```python
from build123d import *

# Parameters (mm, degrees)
SKETCH1_W           = 31.75
SKETCH1_H           = 3.175
BOSS_EXTRUDE1_DEPTH = 31.75
BOSS_EXTRUDE2_DEPTH = 31.75
SKETCH3_W           = 5.08
SKETCH3_H           = 10.541
BOSS_EXTRUDE3_DEPTH = 31.75
SKETCH4_R           = 2.2463125
SKETCH4_R_2         = 2.1193125
CUT_EXTRUDE1_DEPTH  = 31.75
SKETCH6_R           = 2.1193125
BOSS_EXTRUDE4_DEPTH = 15.875
FILLET1_R           = 0.762


with BuildPart() as part:
    # Sketch1 → Boss-Extrude1 (new body)
    with BuildSketch(Plane(origin=(0, 0, 0), x_dir=(1, 0, 0), z_dir=(0, 1, 0))):
        Rectangle(SKETCH1_W, SKETCH1_H)
    extrude(amount=BOSS_EXTRUDE1_DEPTH)

    # Sketch2 → Boss-Extrude2 (add)
    with BuildSketch(Plane(origin=(0, 31.75, 0), x_dir=(1, 0, 0), z_dir=(0, 1, 0))):
        with BuildLine():
            Line((-15.875, 1.5875), (-15.875, 12.3825))
            Line((-15.875, 12.3825), (-10.795, 12.3825))
            ThreePointArc((-10.795, 12.3825), (-7.633217703, 4.749282297), (0, 1.5875))
            Line((0, 1.5875), (-15.875, 1.5875))
        make_face()
    boss_extrude2 = extrude(amount=-BOSS_EXTRUDE2_DEPTH)

    # Mirror1: Boss-Extrude2 across plane
    add(boss_extrude2.mirror(Plane(origin=(0, 0, 0), x_dir=(0, 0, 1), z_dir=(1, 0, 0))))

    # Sketch3 → Boss-Extrude3 (add)
    with BuildSketch(Plane(origin=(0, 31.75, 0), x_dir=(1, 0, 0), z_dir=(0, 1, 0))):
        with Locations((-13.335, 17.653)):
            Rectangle(SKETCH3_W, SKETCH3_H)
    boss_extrude3 = extrude(amount=-BOSS_EXTRUDE3_DEPTH)

    # Mirror2: Boss-Extrude3 across plane
    add(boss_extrude3.mirror(Plane(origin=(0, 0, 0), x_dir=(0, 0, 1), z_dir=(1, 0, 0))))

    # Sketch4 → Cut-Extrude1 (cut)
    with BuildSketch(Plane.XY.offset(1.5875)):
        with Locations((0, 26.035)):
            Circle(SKETCH4_R)
        with Locations((0, 5.715)):
            Circle(SKETCH4_R_2)
    extrude(amount=-CUT_EXTRUDE1_DEPTH, mode=Mode.SUBTRACT)

    # Sketch6 → Boss-Extrude4 (add)
    with BuildSketch(Plane.XY.offset(1.5875)):
        with Locations((0, 5.715)):
            Circle(SKETCH6_R)
    extrude(amount=-BOSS_EXTRUDE4_DEPTH)

    # Fillet1
    fillet1_edges = [part.edges().sort_by_distance(p)[0] for p in [
        (-2.1193125, 5.715, -14.2875),
    ]]
    fillet(fillet1_edges, radius=FILLET1_R)


solid = part.part
```
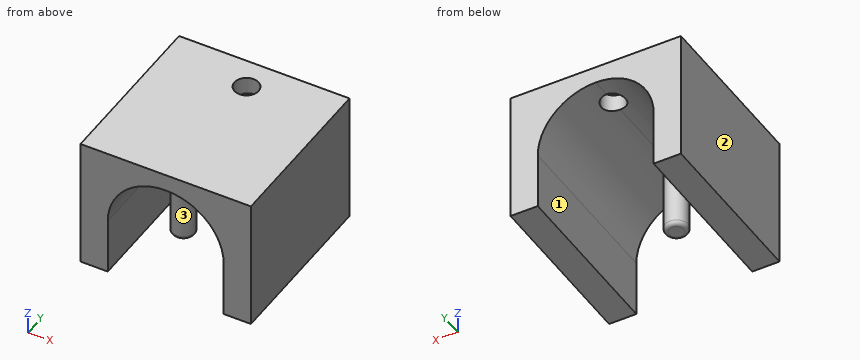
For this review, take the finished solid that the model builds, in its own axes (mm). Face numbers are marked on the shaded views. A direction names the side the tool comes from. Coordinates: 2 decimals unless noted, no trailing zeros. Loops run counter-clockwise (first coordinate to the right, second up) from the corner with the lowest first, then second, coordinate; pieces in that order, holes last. Notation, with made-up numbers: (-39.75, 27.25) - (-4.75, 27.25) arc R17 ccw to (-4.75, 52.25) - close; hole circle Ø3 at (41, 47.25). An arc over 180 degrees is marked (long way). Use one line per item in the form item = value. Start each with the question number.
1) For pin 1 (1.4 mm diameter, centred on x = 0.5, y = 6, fed in from -Z); pin 2 (7 mm diameter, centred on x = 0, y = 26.035, fed in from -Z); pin 3 (8 mm diameter, centred on x = 5, z = -19, fed in from -Y), all flat-tipped, find the tip position at first contact; note any pin that passes through.
2) To check wall thickness, follow probe 1 along Y at (x, z) = (0, -0.5); probe 2 along X at (y, z) = (2, -21) (3 decimals); probe 3 along X at (y, z) = (4, -9.75) (3 decimals). State the ranges of each line that lie inside material, in increasing order. Write a range as from..to.
3) Take a section at C-C (z = -8.75). State the section outline as (x, y) points (3 decimals), plus the area to 3 significant figures.
4) Take a section at B-B (y = 20). State the section outline as (x, z) points (1 decimal), plus the area to 3 significant figures.
5) Take a section at A-A (z = -18.25). State the section outline as (x, y) points (3 decimals), plus the area to 3 significant figures.
6) Take a section at D-D (z = -3.75). State the section outline as (x, y) points (3 decimals).
7) For the marked faces 1, 2 and 3, list the 3-axis set-ups (+Z, -Z, +X, -X, +Y, -Y) from which the entire face can be reached by the end or side of a thin tool; tool diameter is ignored.
From the geometry:
q1.pin_1 = -14.29
q1.pin_2 = -2.17
q1.pin_3 = through
q2.probe_1 = 0..23.79, 28.28..31.75
q2.probe_2 = -15.875..-10.795, 10.795..15.875
q2.probe_3 = -15.875..-10.469, -1.245..1.245, 10.469..15.875
q3.outline = (-15.875, 0) - (-10.165, 0) - (-10.165, 31.75) - (-15.875, 31.75) - close; circle Ø4.239 at (0, 5.715); (10.165, 0) - (15.875, 0) - (15.875, 31.75) - (10.165, 31.75) - close
q3.area = 377 mm2
q4.outline = (-15.9, -22.9) - (-10.8, -22.9) - (-10.8, -12.4) arc R10.8 cw to (10.8, -12.4) - (10.8, -22.9) - (15.9, -22.9) - (15.9, 1.6) - (-15.9, 1.6) - close
q4.area = 368 mm2
q5.outline = (-15.875, 0) - (-10.795, 0) - (-10.795, 31.75) - (-15.875, 31.75) - close; (10.795, 0) - (15.875, 0) - (15.875, 31.75) - (10.795, 31.75) - close
q5.area = 323 mm2
q6.outline = (-15.875, 0) - (-6.482, 0) - (-6.482, 31.75) - (-15.875, 31.75) - close; circle Ø4.239 at (0, 5.715); (6.482, 0) - (15.875, 0) - (15.875, 31.75) - (6.482, 31.75) - close
q7.face_1 = -Z, +Y, -Y
q7.face_2 = +Z, -Z, -X, +Y, -Y
q7.face_3 = -Z
